```python
from build123d import *

# Parameters (mm, degrees)
SKETCH_1_W      = 400
SKETCH_1_H      = 400
EXTRUDE_1_DEPTH = 200
SKETCH_2_R      = 12.5
EXTRUDE_2_DEPTH = 50
FILLET_1_R      = 10
SHELL_1_T       = -5


with BuildPart() as part:
    # 스케치1 → 보스-돌출1 (new body)
    with BuildSketch(Plane.XY):
        with Locations((200, -200)):
            Rectangle(SKETCH_1_W, SKETCH_1_H)
    extrude(amount=EXTRUDE_1_DEPTH)

    # 스케치2 → 보스-돌출2 (add)
    with BuildSketch(Plane.XY.offset(200)):
        with Locations((200, -198.566815637)):
            Circle(SKETCH_2_R)
    extrude(amount=EXTRUDE_2_DEPTH)

    # 필렛1
    fillet_1_edges = [part.edges().sort_by_distance(p)[0] for p in [
        (400, -200, 200),
        (200, 0, 200),
        (187.5, -198.566815637, 200),
        (0, -200, 200),
        (200, 0, 0),
        (400, -200, 0),
        (200, -400, 0),
        (0, -200, 0),
        (200, -400, 200),
        (0, 0, 100),
        (400, 0, 100),
        (400, -400, 100),
        (0, -400, 100),
    ]]
    fillet(fillet_1_edges, radius=FILLET_1_R)

    # 쉘1
    shell_1_openings = [part.faces().sort_by_distance(p)[0] for p in [
        (200, -198.566815637, 250),
    ]]
    offset(amount=SHELL_1_T, openings=shell_1_openings, kind=Kind.INTERSECTION)


solid = part.part
```
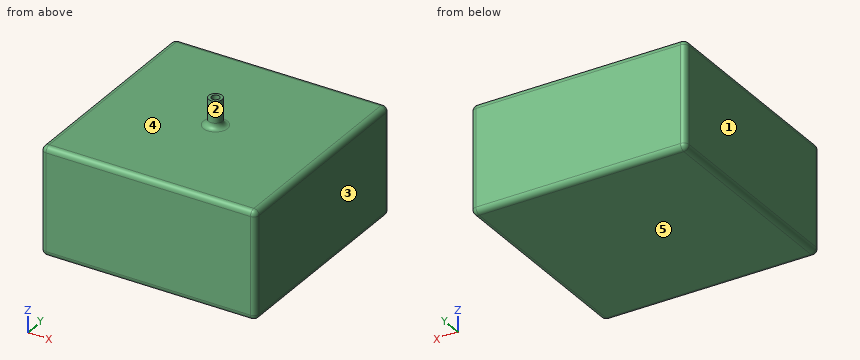
Geometry check sheet. Reference: the model listing, model coordinates, mm. Face numbers are marked on the shaded views. A direction names the side the tool comes from. Give positions to 0.01 mm unless a question says otherwise; leave off trailing zeros. Order: outer loops, then holes, each group sorted by start corner. A loop starts at its lowest first (then second) coordinate and runs counter-clockwise, first axis right, second up. Notation, with made-up numbers: (82, -31.75) -> (120, -31.75) arc R26 ccw to (120, 6.25) -> close; hole circle Ø6 at (36.25, -32.75). An arc over 180 degrees is marked (long way). Write each question's results on one line, items separated by ' | '. Start each with the question number.
(1) Sectioned sample at C-C (x = 200). Enter the section's corners in (y, z).
(2) Mould release check, pull along Z, two halves, no side actions. Record for the marked faces 3, 4 and 5: pulls with the +Z half, pulls with the -Z half, needs draft (parallel to the pull), parting line crosses it, or undercut.
(3) Sectioned sample at B-B (z = 50.5). Enter the section's corners in (x, y).
(4) Access from +Z, -Z, +X, -X, +Y, -Y to the whole of each face (thin tool, end or side, straight path). Record for the marked faces 1 and 2.
(5) Scan lines: line 1 (Z direction, x = 219.5, y = -294.5); line 2 (X direction, y = -295, z = 121.5); line 3 (Y direction, x = 200, z = 229). Record each from-to range of solid material in increasing order.
(6) Sectioned sample at A-A (x = 263.5). Enter the section's corners in (y, z).
Answer below:
1) outline: (-400, 10) arc R10 ccw to (-390, 0) -> (-10, 0) arc R10 ccw to (0, 10) -> (0, 190) arc R10 ccw to (-10, 200) -> (-176.07, 200) arc R10 cw to (-186.07, 210) -> (-186.07, 250) -> (-191.07, 250) -> (-191.07, 210) arc R15 ccw to (-176.07, 195) -> (-10, 195) arc R5 cw to (-5, 190) -> (-5, 10) arc R5 cw to (-10, 5) -> (-390, 5) arc R5 cw to (-395, 10) -> (-395, 190) arc R5 cw to (-390, 195) -> (-221.07, 195) arc R15 ccw to (-206.07, 210) -> (-206.07, 250) -> (-211.07, 250) -> (-211.07, 210) arc R10 cw to (-221.07, 200) -> (-390, 200) arc R10 ccw to (-400, 190) -> close
2) face 3: needs draft | face 4: pulls with the +Z half | face 5: pulls with the -Z half
3) outline: (0, -390) arc R10 ccw to (10, -400) -> (390, -400) arc R10 ccw to (400, -390) -> (400, -10) arc R10 ccw to (390, 0) -> (10, 0) arc R10 ccw to (0, -10) -> close; hole (5, -390) arc R5 ccw to (10, -395) -> (390, -395) arc R5 ccw to (395, -390) -> (395, -10) arc R5 ccw to (390, -5) -> (10, -5) arc R5 ccw to (5, -10) -> close
4) face 1: +Z, -Z, -X, +Y, -Y | face 2: +Z
5) line 1: 0 to 5, 195 to 200 | line 2: 0 to 5, 395 to 400 | line 3: -211.07 to -206.07, -191.07 to -186.07
6) outline: (-400, 10) arc R10 ccw to (-390, 0) -> (-10, 0) arc R10 ccw to (0, 10) -> (0, 190) arc R10 ccw to (-10, 200) -> (-390, 200) arc R10 ccw to (-400, 190) -> close; hole (-395, 10) arc R5 ccw to (-390, 5) -> (-10, 5) arc R5 ccw to (-5, 10) -> (-5, 190) arc R5 ccw to (-10, 195) -> (-390, 195) arc R5 ccw to (-395, 190) -> close
